```python
from build123d import *

# Parameters (mm, degrees)
BOSS_EXTRUDE1_DEPTH = 4.7625
CHAMFER1_SIZE       = 1.5875
CHAMFER1_SIZE2      = 12.7
CHAMFER2_SIZE       = 1.5875
CHAMFER2_SIZE2      = 12.7


with BuildPart() as part:
    # Sketch1 → Boss-Extrude1 (new body)
    with BuildSketch(Plane.XY):
        Polygon((0, 0), (254, 0), (228.6, 127), (177.8, 127), align=None)
    extrude(amount=BOSS_EXTRUDE1_DEPTH)

    # Chamfer1
    chamfer1_edges = [part.edges().sort_by_distance(p)[0] for p in [
        (88.9, 63.5, 4.7625),
        (88.9, 63.5, 0),
    ]]
    chamfer1_side = [part.faces().sort_by_distance(p)[0] for p in [
        (88.9, 63.5, 2.38125),
    ]]
    chamfer(chamfer1_edges, length=CHAMFER1_SIZE, length2=CHAMFER1_SIZE2, reference=chamfer1_side[0])

    # Chamfer2
    chamfer2_edges = [part.edges().sort_by_distance(p)[0] for p in [
        (241.3, 63.5, 4.7625),
        (241.3, 63.5, 0),
    ]]
    chamfer2_side = [part.faces().sort_by_distance(p)[0] for p in [
        (241.3, 63.5, 2.38125),
    ]]
    chamfer(chamfer2_edges, length=CHAMFER2_SIZE, length2=CHAMFER2_SIZE2, reference=chamfer2_side[0])


solid = part.part
```
Build history of the part. All positions in model axes, mm. Give positions to 0.01 mm unless a question says otherwise; leave off trailing zeros. Loops run counter-clockwise (first coordinate to the right, second up) from the corner with the lowest first, then second, coordinate; pieces in that order, holes last. Notation, with made-up numbers: (9, -29.75) - (63, -29.75) arc R21 ccw to (63, -9.75) - close; hole circle Ø10 at (49.5, 7.5). An arc over 180 degrees is marked (long way). Use a Markdown table: item, result.
(1) Band-saw the part on A-A (y = 62.5). Give the cut face in (x, z) (1 decimal), and give its area (3 significant figures).
Taken from the geometry:
| item | result |
|---|---|
| outline | (87.5, 1.6) - (109.3, 0) - (228.5, 0) - (241.5, 1.6) - (241.5, 3.2) - (228.5, 4.8) - (109.3, 4.8) - (87.5, 3.2) - close |
| area | 678 mm2 |
(2) Band-saw the part on C-C (z = 0.8). Give the cut face in (x, y).
Taken from the geometry:
| item | result |
|---|---|
| outline | (10.84, 0) - (247.58, 0) - (222.18, 127) - (188.64, 127) - close |
(3) Band-saw the part on B-B (x = 146). Give the cut face in (y, z) (1 decimal).
Taken from the geometry:
| item | result |
|---|---|
| outline | (0, 0) - (88.7, 0) - (104.3, 1.6) - (104.3, 3.2) - (88.7, 4.8) - (0, 4.8) - close |
(4) Drop a flat-ended pin along its axis: pin 1 Ø2 at (x, z) = (79.5, 1.5) entering from +Y. Give the stop position or say it passes through.
Taken from the geometry:
| item | result |
|---|---|
| pin 1 | y = 57.5 |
(5) Wall check: line 1 along X through (y, z) = (11, 2.5); line 2 along X through (y, z) = (28, 2.65); line 3 along Y through (x, z) = (77.5, 2.1). Give the ranges that are in metal, low to high.
Taken from the geometry:
| item | result |
|---|---|
| line 1 | 15.4 to 251.8 |
| line 2 | 39.2 to 248.4 |
| line 3 | 0 to 55.36 |
(6) Band-saw the part on D-D (y = 25). Give the cut face in (x, z) (1 decimal).
Taken from the geometry:
| item | result |
|---|---|
| outline | (35, 1.6) - (56.8, 0) - (236, 0) - (249, 1.6) - (249, 3.2) - (236, 4.8) - (56.8, 4.8) - (35, 3.2) - close |
